Build history of the part. All positions in model axes, mm. A direction names the side the tool comes from. Give positions to 0.01 mm unless a question says otherwise; leave off trailing zeros. Order: outer loops, then holes, each group sorted by start corner. A loop starts at its lowest first (then second) coordinate and runs counter-clockwise, first axis right, second up. Notation, with made-up numbers: (-23, -28) -> (-19, -28) arc R31 cw to (-19, 11) -> close; hole circle Ø2 at (6.25, 66.25). An arc over 180 degrees is marked (long way). One line per item, written item: value. Start each with the question number.
(1) Probe line 1 (X direction, y = -15, z = -254); line 2 (Y direction, x = -59, z = -456); line 3 (Z direction, x = 105, y = 51.5). List the from-to ranges inside material, lowest first.
(2) Two-plate mould, pull along X, no slides. Class faces 4 (the flat face through (65, 208.545, -296)), 5 (the flat face through (65, 203.545, -293)), 6 (the flat face through (267.482, 6, -296)), 7 (the flat face through (65, -186.455, -293)): +X half, -X half, draft (parallel to the pull), parting line (faces both ways), or undercut.
(3) Saw through at A-A on z = -329.5. Give the cut face in (x, y).
(4) Which spindle directions (+Z, -Z, +X, -X, +Y, -Y) get a long thin tool onto all of the face, cutting with end or side? Do faces 1 (the flat face through (65, 11, -600)), 2 (the cylindrical face through (265.017, 5.29, -525.213)), 3 (the flat face through (-127.518, 6, -293)). Say none if no direction does.
(5) Saw through at D-D on z = -550. Give the cut face in (x, y).
(6) Saw through at B-B on x = 86.5. Give the cut face in (y, z), plus the area to 3 significant figures.
(7) Saw through at C-C on y = -161.5. Give the cut face in (x, z).
```python
from build123d import *

# Parameters (mm, degrees)
F0_W     = 400
F0_H     = 400
F1_DEPTH = 600
F2_T     = -5
F3_R     = 25
F4_DEPTH = 30


with BuildPart() as f1:
    # F0 (on Top) → F1 (new body)
    with BuildSketch(Plane.XY):
        with Locations((67.481734, 8.544586)):
            Rectangle(F0_W, F0_H)
    extrude(amount=-F1_DEPTH)

    # F2
    f2_openings = [f1.faces().sort_by_distance(p)[0] for p in [
        (67.481734, 8.544586, 0),
    ]]
    offset(amount=F2_T, openings=f2_openings)

    # F3 (on face) → F4 (cut)
    with BuildSketch(Plane.YZ.offset(267.481734)):
        with Locations((8.544586, -550)):
            Circle(F3_R)
    extrude(amount=-F4_DEPTH, mode=Mode.SUBTRACT)


solid = f1.part
```
Results below:
1. line 1: x = -132.52 to -127.52, 262.48 to 267.48
1. line 2: y = -191.46 to -186.46, 203.54 to 208.54
1. line 3: z = -600 to -595
2. face 4: draft
2. face 5: undercut
2. face 6: +X half
2. face 7: undercut
3. outline: (-132.52, -191.46) -> (267.48, -191.46) -> (267.48, 208.54) -> (-132.52, 208.54) -> close; hole (-127.52, -186.46) -> (262.48, -186.46) -> (262.48, 203.54) -> (-127.52, 203.54) -> close
4. face 1: -Z, +X, -X, +Y, -Y
4. face 2: +X
4. face 3: +Z
5. outline: (-132.52, -191.46) -> (267.48, -191.46) -> (267.48, -16.46) -> (262.48, -16.46) -> (262.48, -186.46) -> (-127.52, -186.46) -> (-127.52, 203.54) -> (262.48, 203.54) -> (262.48, 33.54) -> (267.48, 33.54) -> (267.48, 208.54) -> (-132.52, 208.54) -> close
6. outline: (-191.46, -600) -> (208.54, -600) -> (208.54, 0) -> (203.54, 0) -> (203.54, -595) -> (-186.46, -595) -> (-186.46, 0) -> (-191.46, 0) -> close
6. area: 7,950 mm²
7. outline: (-132.52, -600) -> (267.48, -600) -> (267.48, 0) -> (262.48, 0) -> (262.48, -595) -> (-127.52, -595) -> (-127.52, 0) -> (-132.52, 0) -> close
